Input: part model. Units: mm. Frame: model coordinates. A direction names the side the tool comes from. Coordinates: 2 decimals unless noted, no trailing zeros. Order: outer loops, then holes, each group sorted by start corner. A loop starts at its lowest first (then second) coordinate and runs counter-clockwise, first axis right, second up. Notation, with made-up numbers: (39.5, 59.5) - (44.5, 59.5) arc R28 cw to (44.5, 95.5) - close; hole circle Ø6 at (25, -37.75). An arc over 180 degrees is marked (long way). Answer as CSV lines item,"result". Start each with the question number.
Item 1: Section C-C (x = 17.5). Output: boundary loops of the cut face in (y, z), and give its area (3 significant figures).
Item 2: Section B-B (x = 25). Output: boundary loops of the cut face in (y, z), and give its area (3 significant figures).
Item 3: Section D-D (y = 51). Output: boundary loops of the cut face in (x, z).
Item 4: First-contact query: pin 1 (1 mm diameter, centred on x = 24.5, y = 73.5, fed in from +Z); pin 2 (17.5 mm diameter, centred on x = 19, y = 59, fed in from -Z). Flat tips, straight axial feed; report the tip coordinate or a pass-through.
Item 5: Access query for faces 1 (the flat face through (17, 56, -50)), 2 (the flat face through (17, 8, -21)), 3 (the flat face through (17, 118, -68)). Directions: +Z, -Z, +X, -X, +Y, -Y. A direction counts if a zero-diameter tool reaches every point of the face in a straight line with its end or side. Return the directions, or none.
Item 6: Section A-A (z = -19). Output: boundary loops of the cut face in (x, y).
Item 7: Draft query along X for faces 4 (the cylindrical face through (26.69, 4.06, -20.84)), 5 (the flat face through (17, 0, -23)), 6 (the flat face through (35, 59, -45)), 7 (the flat face through (0, 59, -45)). Return one class per face: +X half, -X half, draft (parallel to the pull), parting line (faces both ways), or undercut.
Item 8: Material intervals for line 1 along X through (y, z) = (2, -19); line 2 along Y through (x, z) = (3, -82); line 3 along Z through (x, y) = (28, 81.5), sorted ascending.
from build123d import *

# Parameters (mm, degrees)
BOSS_EXTRUDE1_DEPTH = 35
SKETCH2_R           = 10
CUT_EXTRUDE1_DEPTH  = 10
SKETCH3_R           = 2.5
CUT_EXTRUDE2_DEPTH  = 147.372811683


with BuildPart() as part:
    # Sketch1 → Boss-Extrude1 (new body)
    with BuildSketch(Plane(origin=(0, 0, 0), x_dir=(0, 0, -1), z_dir=(1, 0, 0))):
        with BuildLine():
            Line((0, 0), (0, 4))
            ThreePointArc((0, 4), (1.171572875, 6.828427125), (4, 8))
            Line((4, 8), (38, 8))
            ThreePointArc((38, 8), (40.828427125, 9.171572875), (42, 12))
            Line((42, 12), (42, 114))
            ThreePointArc((42, 114), (43.171572875, 116.828427125), (46, 118))
            Line((46, 118), (90, 118))
            Line((90, 118), (90, 110))
            Line((90, 110), (54, 110))
            ThreePointArc((54, 110), (51.171572875, 108.828427125), (50, 106))
            Line((50, 106), (50, 4))
            ThreePointArc((50, 4), (48.828427125, 1.171572875), (46, 0))
            Line((46, 0), (0, 0))
        make_face()
    extrude(amount=BOSS_EXTRUDE1_DEPTH)

    # Sketch2 → Cut-Extrude1 (cut)
    with BuildSketch(Plane(origin=(0, 118, 0), x_dir=(1, 0, 0), z_dir=(0, 1, 0))):
        with Locations((17.5, 90)):
            Circle(SKETCH2_R)
    extrude(amount=-CUT_EXTRUDE1_DEPTH, mode=Mode.SUBTRACT)

    # Sketch3 → Cut-Extrude2 (cut, through all)
    with BuildSketch(Plane(origin=(0, 8, 0), x_dir=(1, 0, 0), z_dir=(0, 1, 0))):
        with Locations(Location((10, 19, 0), (0, 0, 270))):
            Circle(SKETCH3_R)
        with Locations(Location((25, 19, 0), (0, 0, 270))):
            Circle(SKETCH3_R)
    extrude(amount=-CUT_EXTRUDE2_DEPTH, mode=Mode.SUBTRACT)


solid = part.part
Determined:
1,outline,"(0, -46) arc R4 ccw to (4, -50) - (106, -50) arc R4 cw to (110, -54) - (110, -80) - (118, -80) - (118, -46) arc R4 ccw to (114, -42) - (12, -42) arc R4 cw to (8, -38) - (8, -4) arc R4 ccw to (4, 0) - (0, 0) - close"
1,area,"1,520 mm^2"
2,outline,"(0, -46) arc R4 ccw to (4, -50) - (106, -50) arc R4 cw to (110, -54) - (110, -83.39) - (118, -83.39) - (118, -46) arc R4 ccw to (114, -42) - (12, -42) arc R4 cw to (8, -38) - (8, -21.5) - (0, -21.5) - close; (0, -16.5) - (8, -16.5) - (8, -4) arc R4 ccw to (4, 0) - (0, 0) - close"
2,area,"1,500 mm^2"
3,outline,"(0, -50) - (35, -50) - (35, -42) - (0, -42) - close"
4,pin 1,"stops at z = -42"
4,pin 2,"stops at z = -50"
5,face 1,"-Z, +X, -X, -Y"
5,face 2,"+Z, +X, -X, +Y"
5,face 3,"+Z, -Z, +X, -X, +Y"
6,outline,"(0, 0) - (7.5, 0) - (7.5, 8) - (0, 8) - close; (12.5, 0) - (22.5, 0) - (22.5, 8) - (12.5, 8) - close; (27.5, 0) - (35, 0) - (35, 8) - (27.5, 8) - close"
7,face 4,"undercut"
7,face 5,"draft"
7,face 6,"+X half"
7,face 7,"-X half"
8,line 1,"x = 0 to 7.5, 12.5 to 22.5, 27.5 to 35"
8,line 2,"y = 110 to 118"
8,line 3,"z = -50 to -42"
